from build123d import *

# Parameters (mm, degrees)
SKETCH1_W           = 40
SKETCH1_H           = 40
SKETCH1_W_2         = 34
SKETCH1_H_2         = 34
BOSS_EXTRUDE1_DEPTH = 450
SKETCH2_R           = 4
SKETCH2_R_2         = 20
CUT_EXTRUDE1_DEPTH  = 600


with BuildPart() as part:
    # Sketch1 → Boss-Extrude1 (new body)
    with BuildSketch(Plane.XY):
        with Locations((20, 20)):
            Rectangle(SKETCH1_W, SKETCH1_H)
        with Locations((20, 20)):
            Rectangle(SKETCH1_W_2, SKETCH1_H_2, mode=Mode.SUBTRACT)
    extrude(amount=BOSS_EXTRUDE1_DEPTH)

    # Sketch2 → Cut-Extrude1 (cut)
    with BuildSketch(Plane(origin=(0, 40, 0), x_dir=(1, 0, 0), z_dir=(0, 1, 0))):
        with Locations(Location((20, -399.819329365, 0), (0, 0, 270))):
            Circle(SKETCH2_R)
        with Locations(Location((20, -433.273109788, 0), (0, 0, 270))):
            Circle(SKETCH2_R)
        with Locations((20, 0)):
            Circle(SKETCH2_R_2)
    extrude(amount=-CUT_EXTRUDE1_DEPTH, mode=Mode.SUBTRACT)


solid = part.part
Verification items for the finished model (mm, model axes). A direction names the side the tool comes from. Give positions to 0.01 mm unless a question says otherwise; leave off trailing zeros. Write each loop counter-clockwise with the first axis right and the second up, starting at its lowest first coordinate (ties: lowest second). Pieces come first, ordered by that corner, then holes.
(1) Cross-section at C-C (y = 9.5). Enter the section's corners in (x, z), plus the area to 3 significant figures.
(2) Gauge pin test, flat end, axial feed: pin 1 (10 mm diameter, centred on x = 16.5, y = 6.5, fed in from -Z). Record the tip position at first contact, or that the pin passes through.
(3) Mould release check, pull along Z, two halves, no side actions. Record for faces 1 (the face through (20.176, 1.521, 395.823)), 2 (the face through (2, 20, 450)), 3 (the face through (20, 3, 227)): +Z half, -Z half, draft (parallel to the pull), parting line (faces both ways), or undercut.
(4) Material ranges on line 1 (Y direction, x = 12, z = 383), recorded low to high.
(5) Access from +Z, -Z, +X, -X, +Y, -Y to the whole of each face (thin tool, end or side, straight path). Record for faces 4 (the face through (20, 40, 222)), 5 (the face through (3, 20, 227)).
(6) Cross-section at A-A (x = 20). Enter the section's corners in (y, z).
(7) Cross-section at B-B (z = 157.5). Enter the section's corners in (x, y).
Worked out:
1. outline: (0, 0) arc R20 cw to (3, 10.54) - (3, 450) - (0, 450) - close; (37, 10.54) arc R20 cw to (40, 0) - (40, 450) - (37, 450) - close
1. area: 2,660 mm2
2. pin 1: stops at z = 18.71
3. face 1: undercut
3. face 2: +Z half
3. face 3: draft
4. line 1: y = 0 to 3, 37 to 40
5. face 4: +Z, -Z, +X, -X, +Y
5. face 5: +Z, -Z
6. outline: (0, 20) - (3, 20) - (3, 395.82) - (0, 395.82) - close; (0, 403.82) - (3, 403.82) - (3, 429.27) - (0, 429.27) - close; (0, 437.27) - (3, 437.27) - (3, 450) - (0, 450) - close; (37, 20) - (40, 20) - (40, 395.82) - (37, 395.82) - close; (37, 403.82) - (40, 403.82) - (40, 429.27) - (37, 429.27) - close; (37, 437.27) - (40, 437.27) - (40, 450) - (37, 450) - close
7. outline: (0, 0) - (40, 0) - (40, 40) - (0, 40) - close; hole (3, 3) - (37, 3) - (37, 37) - (3, 37) - close
